```python
from build123d import *

# Parameters (mm, degrees)
BOSS_EXTRU_1_DEPTH      = 10
ESQUISSE4_W             = 70
ESQUISSE4_H             = 80
BOSS_EXTRU_2_DEPTH      = 10
BOSS_EXTRU_3_DEPTH      = 10
ESQUISSE7_R             = 12.5
ENL_V_MAT_EXTRU_2_DEPTH = 155.677082983
BOSS_EXTRU_4_DEPTH      = 10
ESQUISSE10_R            = 10
ENL_V_MAT_EXTRU_3_DEPTH = 219.746428542
CONG_1_R                = 5
CONG_5_R                = 12
CONG_6_R                = 12
CONG_7_R                = 3
CONG_8_R                = 3


with BuildPart() as part:
    # Esquisse1 → Boss.-Extru.1 (new body)
    with BuildSketch(Plane.XY):
        with BuildLine():
            Line((0, 0), (0, 60))
            ThreePointArc((0, 60), (35, 95), (70, 60))
            Line((70, 60), (70, 0))
            Line((70, 0), (0, 0))
        make_face()
    extrude(amount=BOSS_EXTRU_1_DEPTH)

    # Esquisse4 → Boss.-Extru.2 (add)
    with BuildSketch(Plane(origin=(0, 0, 0), x_dir=(-1, 0, 0), z_dir=(0, -1, 0))):
        with Locations((-35, -50)):
            Rectangle(ESQUISSE4_W, ESQUISSE4_H)
    extrude(amount=-BOSS_EXTRU_2_DEPTH)

    # Esquisse6 → Boss.-Extru.3 (add)
    with BuildSketch(Plane.XY.offset(90)):
        with BuildLine():
            Line((0, 0), (0, 60))
            ThreePointArc((0, 60), (35, 95), (70, 60))
            Line((70, 60), (70, 0))
            Line((70, 0), (0, 0))
        make_face()
    extrude(amount=BOSS_EXTRU_3_DEPTH)

    # Esquisse7 → Enlèv. mat.-Extru.2 (cut, through all)
    with BuildSketch(Plane.XY.offset(100)):
        with Locations((35, 60)):
            Circle(ESQUISSE7_R)
    extrude(amount=-ENL_V_MAT_EXTRU_2_DEPTH, mode=Mode.SUBTRACT)

    # Esquisse9 → Boss.-Extru.4 (add)
    with BuildSketch(Plane(origin=(0, 10, 0), x_dir=(1, 0, 0), z_dir=(0, 1, 0))):
        with BuildLine():
            Line((70, -25), (150, -25))
            ThreePointArc((150, -25), (175, -50), (150, -75))
            Line((150, -75), (70, -75))
            Line((70, -75), (70, -25))
        make_face()
    extrude(amount=-BOSS_EXTRU_4_DEPTH)

    # Esquisse10 → Enlèv. mat.-Extru.3 (cut, through all)
    with BuildSketch(Plane(origin=(0, 10, 0), x_dir=(1, 0, 0), z_dir=(0, 1, 0))):
        with Locations(Location((150, -50, 0), (0, 0, 180))):
            Circle(ESQUISSE10_R)
        with Locations(Location((100, -50, 0), (0, 0, 180))):
            Circle(ESQUISSE10_R)
    extrude(amount=-ENL_V_MAT_EXTRU_3_DEPTH, mode=Mode.SUBTRACT)

    # Congé1
    cong_1_edges = [part.edges().sort_by_distance(p)[0] for p in [
        (70, 5, 75),
        (70, 5, 25),
    ]]
    fillet(cong_1_edges, radius=CONG_1_R)

    # Congé5
    cong_5_edges = [part.edges().sort_by_distance(p)[0] for p in [
        (35, 0, 100),
    ]]
    fillet(cong_5_edges, radius=CONG_5_R)

    # Congé6
    cong_6_edges = [part.edges().sort_by_distance(p)[0] for p in [
        (35, 0, 0),
    ]]
    fillet(cong_6_edges, radius=CONG_6_R)

    # Congé7
    cong_7_edges = [part.edges().sort_by_distance(p)[0] for p in [
        (35, 10, 10),
    ]]
    fillet(cong_7_edges, radius=CONG_7_R)

    # Congé8
    cong_8_edges = [part.edges().sort_by_distance(p)[0] for p in [
        (35, 10, 90),
    ]]
    fillet(cong_8_edges, radius=CONG_8_R)


solid = part.part
```
Can you work these out from the model? Positions are in its coordinate system, mm. A direction names the side the tool comes from. Coordinates: 2 decimals unless noted, no trailing zeros. Write each loop counter-clockwise with the first axis right and the second up, starting at its lowest first coordinate (ties: lowest second). Pieces come first, ordered by that corner, then holes. Notation, with made-up numbers: M 83.25,84 L 96.25,84 A38 cw 96.25,122 Z; hole C 3,-19.5 d4. An arc over 180 degrees is marked long. Answer as CSV lines item,"result".
Item 1: Imagine slicing it at D-D on x = 100. List the corners of the cut face in (y, z) for me, plus the area to 3 significant figures.
Geometry results:
outline,"M 0,25 L 10,25 L 10,40 L 0,40 Z; M 0,60 L 10,60 L 10,75 L 0,75 Z"
area,"300 mm2"
Item 2: Imagine slicing it at B-B on z = 50. List the corners of the cut face in (x, y) for me.
Geometry results:
outline,"M 0,0 L 90,0 L 90,10 L 0,10 Z; M 110,0 L 140,0 L 140,10 L 110,10 Z; M 160,0 L 175,0 L 175,10 L 160,10 Z"
Item 3: Imagine slicing it at A-A on x = 35. List the corners of the cut face in (y, z) for me, plus the area to 3 significant figures.
Geometry results:
outline,"M 0,12 A12 ccw 12,0 L 47.5,0 L 47.5,10 L 13,10 A3 cw 10,13 L 10,87 A3 cw 13,90 L 47.5,90 L 47.5,100 L 12,100 A12 ccw 0,88 Z; M 72.5,0 L 95,0 L 95,10 L 72.5,10 Z; M 72.5,90 L 95,90 L 95,100 L 72.5,100 Z"
area,"2,140 mm2"
Item 4: On a 3-axis mill with a long thin cutter (end or side, diameter ignored), from which of +Z, -Z, +X, -X, +Y, -Y can I reach the whole of each face in a straight line? I mean faces 1 (the flat face through (69, 10, 49)), 2 (the flat face through (70, 30, 5)), 3 (the cylindrical face through (25.79, 68.45, 95.07)). Say none if no direction works.
Geometry results:
face 1,"+X, -X, +Y"
face 2,"-Z, +X, +Y, -Y"
face 3,"+Z, -Z"
Item 5: Please list where these lines run through material, in increasing order: line 1 along Z through (x, y) = (100, 8); line 2 along Z through (x, y) = (8, 44); line 3 along Y through (x, z) = (37, 69).
Geometry results:
line 1,"z = 25 to 40, 60 to 75"
line 2,"z = 0 to 10, 90 to 100"
line 3,"y = 0 to 10"
Item 6: I'm going to push flat-ended pins straight in: P1, Ø18, axis at x = 150, z = 50, coming from the -Y side; P2, Ø16, axis at y = 15.5, z = 85.5, coming from the +X side; P3, Ø3, axis at x = 111, y = 5.5, coming from the +Z side; P4, Ø3, axis at x = 113.5, y = 3, coming from the -Z side. Where does each tip first touch, or does it pass through?
Geometry results:
P1,"passes through"
P2,"stops at x = 70.01"
P3,"stops at z = 75"
P4,"stops at z = 25"
Item 7: Imagine slicing it at C-C on y = 26. List the corners of the cut face in (x, z) for me.
Geometry results:
outline,"M 0,0 L 70,0 L 70,10 L 0,10 Z; M 0,90 L 70,90 L 70,100 L 0,100 Z"
Item 8: We'd pull the mould along Z, two halves only. Please class faces 4 (the cylindrical face through (71, 5, 77)), 5 (the flat face through (35, 45, 90)), 6 (the cylindrical face through (34.23, 94.99, 94.93)): +Z half, -Z half, draft (parallel to the pull), parting line (faces both ways), or undercut.
Geometry results:
face 4,"+Z half"
face 5,"undercut"
face 6,"draft"
